For this review, take the finished solid that the model builds, in its own axes (mm). A direction names the side the tool comes from. Give positions to 0.01 mm unless a question says otherwise; leave off trailing zeros. Write each loop counter-clockwise with the first axis right and the second up, starting at its lowest first coordinate (ties: lowest second). Pieces come first, ordered by that corner, then holes. Notation, with made-up numbers: M 21,-32 L 78,-32 A20 cw 78,6 Z; hole C 6.5,0 d11. An arc over 180 degrees is marked long. Write item = value, one per line.
```python
from build123d import *

# Parameters (mm, degrees)
F0_R     = 7.5
F1_DEPTH = 1
F2_R     = 5.9
F3_DEPTH = 4
F4_R     = 2
F5_DEPTH = 25


with BuildPart() as f1:
    # F0 (on Top) → F1 (new body)
    with BuildSketch(Plane.XY):
        with Locations((-54.880984, -32.195751)):
            Circle(F0_R)
    extrude(amount=F1_DEPTH)

    # F2 (on face) → F3 (join)
    with BuildSketch(Plane.XY.offset(1)):
        with Locations((-54.880984, -32.195751)):
            Circle(F2_R)
    extrude(amount=F3_DEPTH)

    # F4 (on face) → F5 (cut)
    with BuildSketch(Plane.XY.offset(5)):
        with Locations((-54.880984, -32.195751)):
            Circle(F4_R)
    extrude(amount=-F5_DEPTH, mode=Mode.SUBTRACT)


solid = f1.part
```
1. We need section A-A, the plane x = -53.75. Write out the cut boundary in (y, z), then the cut area to 3 significant figures.
Responses:
outline = M -39.61,0 L -33.85,0 L -33.85,5 L -37.99,5 L -37.99,1 L -39.61,1 Z; M -30.55,0 L -24.78,0 L -24.78,1 L -26.41,1 L -26.41,5 L -30.55,5 Z
area = 44.7 mm2
2. Machinability: for faces 1 (the face through (-60.775, -31.936, 2.972)), 2 (the face through (-55, -35, 5)), which of the approach directions +Z, -Z, +X, -X, +Y, -Y give a long, thin tool a straight path to every point of the face, cutting with its end or side? Answer none if there is none.
Responses:
face_1 = +Z
face_2 = +Z, +X, -X, +Y, -Y
3. For line 1 along Z through (x, y) = (-49.75, -28.25); line 2 along X through (y, z) = (-34, 3.55); line 3 along X through (y, z) = (-31.5, 1.15), list the stretches that pass through material, from the lowest coordinate up. Write a range as from..to.
Responses:
line_1 = 0..1
line_2 = -60.5..-55.74, -54.02..-49.26
line_3 = -60.74..-56.76, -53.01..-49.02
4. The part is to be moulded in two halves that separate along Y. For faces 3 (the face through (-60.41, -27.13, 0.49)), 4 (the face through (-56.88, -32.11, 2.54)), 5 (the face through (-54.9, -38.3, 1)), say which applies: +Y half, -Y half, draft (parallel to the pull), parting line (faces both ways), or undercut.
Responses:
face_3 = parting line
face_4 = undercut
face_5 = draft
5. We need section B-B, the plane y = -27.5. Write out the cut boundary in (x, z).
Responses:
outline = M -60.73,0 L -49.03,0 L -49.03,1 L -51.31,1 L -51.31,5 L -58.45,5 L -58.45,1 L -60.73,1 Z
6. We need section D-D, the plane z = 3.9. Write out the cut boundary in (x, y), then the cut area to 3 significant figures.
Responses:
outline = C -54.88,-32.2 d11.8; hole C -54.88,-32.2 d4
area = 96.8 mm2
7. We need section C-C, the plane x = -51.25. Write out the cut boundary in (y, z).
Responses:
outline = M -38.76,0 L -25.63,0 L -25.63,1 L -27.55,1 L -27.55,5 L -36.85,5 L -36.85,1 L -38.76,1 Z
